```python
from build123d import *

# Parameters (mm, degrees)
SKETCH2_W           = 90
SKETCH2_H           = 150
BOSS_EXTRUDE1_DEPTH = 20
BOSS_EXTRUDE2_DEPTH = 70
FILLET1_R           = 10
SKETCH4_R           = 41.5
BOSS_EXTRUDE3_DEPTH = 35


with BuildPart() as part:
    # Sketch2 → Boss-Extrude1 (new body)
    with BuildSketch(Plane(origin=(0, 0, 0), x_dir=(1, 0, 0), z_dir=(0, 1, 0))):
        Rectangle(SKETCH2_W, SKETCH2_H)
    extrude(amount=BOSS_EXTRUDE1_DEPTH)

    # Sketch3 → Boss-Extrude2 (add)
    with BuildSketch(Plane(origin=(0, 20, 0), x_dir=(1, 0, 0), z_dir=(0, 1, 0))):
        with BuildLine():
            Line((-45, 75), (45, 75))
            Line((45, 75), (45, -121.380973526))
            ThreePointArc((45, -121.380973526), (65.777396776, -198.944395449), (0, -245))
            Line((0, -245), (-70, -245))
            Line((-70, -245), (-70, -175))
            ThreePointArc((-70, -175), (-63.442887702, -145.419601085), (-45, -121.380973526))
            Line((-45, -121.380973526), (-45, 75))
        make_face()
    extrude(amount=BOSS_EXTRUDE2_DEPTH)

    # Fillet1
    fillet1_edges = [part.edges().sort_by_distance(p)[0] for p in [
        (-70, 55, 245),
    ]]
    fillet(fillet1_edges, radius=FILLET1_R)

    # Sketch4 → Boss-Extrude3 (add)
    with BuildSketch(Plane(origin=(0, 0, -75), x_dir=(-1, 0, 0), z_dir=(0, 0, -1))):
        with Locations((0, 48.5)):
            Circle(SKETCH4_R)
    extrude(amount=BOSS_EXTRUDE3_DEPTH)


solid = part.part
```
Input: part model. Units: mm. Frame: model coordinates. A direction names the side the tool comes from. Give positions to 0.01 mm unless a question says otherwise; leave off trailing zeros. Order: outer loops, then holes, each group sorted by start corner. A loop starts at its lowest first (then second) coordinate and runs counter-clockwise, first axis right, second up.
1. Section C-C on z = -38. Return the cut outline in (x, y).
Derived:
outline: (-45, 0) - (45, 0) - (45, 90) - (-45, 90) - close
2. Material intervals for L1, parallel to Y at x = 25.5, z = 90; L2, parallel to X at y = 80.5, z = -15; L3, parallel to Z at x = -23, y = 8, sorted ascending.
Derived:
L1: y = 20 to 90
L2: x = -45 to 45
L3: z = -75 to 75
3. Section D-D on x = 6.5. Return the cut outline in (y, z), and give its area (3 significant figures).
Derived:
outline: (0, -75) - (7.51, -75) - (7.51, -110) - (89.49, -110) - (89.49, -75) - (90, -75) - (90, 244.7) - (20, 244.7) - (20, 75) - (0, 75) - close
area: 28,200 mm2
4. Section A-A on y = 43. Return the cut outline in (x, z), and give its area (3 significant figures).
Derived:
outline: (-70, 175) arc R70 ccw to (-45, 121.38) - (-45, -75) - (-41.13, -75) - (-41.13, -110) - (41.13, -110) - (41.13, -75) - (45, -75) - (45, 121.38) arc R70 ccw to (0, 245) - (-60, 245) arc R10 ccw to (-70, 235) - close
area: 36,000 mm2
5. Reachability of faces 1 (the flat face through (1, 49, -110)), 2 (the flat face through (1, 20, 159)), 3 (the flat face through (45, 44, 22)), 4 (the flat face through (-45, 44, 25)), 5 (the cylindrical face through (8.996, 7.987, -92.255)) from +Z, -Z, +X, -X, +Y, -Y: full face, straight path, thin tool, end or side. Return the list, or none.
Derived:
face 1: -Z, +X, -X, +Y, -Y
face 2: +Z, +X, -X, -Y
face 3: -Z, +X, +Y, -Y
face 4: -Z, -X, +Y, -Y
face 5: -Z
6. Section B-B on x = -17. Return the cut outline in (y, z).
Derived:
outline: (0, -75) - (10.64, -75) - (10.64, -110) - (86.36, -110) - (86.36, -75) - (90, -75) - (90, 245) - (20, 245) - (20, 75) - (0, 75) - close
7. Pin query (flat end, axial travel): pin 1 (6 mm diameter, centred on x = 38, y = 43, fed in from +Z); pin 2 (3 mm diameter, centred on y = 45, z = 125.5, fed in from -X); pin 3 (3 mm diameter, centred on y = 57.5, z = -37.5, fed in from +X). Return the tip coordinate at first contact, or that it passes through.
Derived:
pin 1: stops at z = 235.62
pin 2: stops at x = -50.95
pin 3: stops at x = 45
